from build123d import *

# Parameters (mm, degrees)
F0_W     = 914.4
F0_H     = 330.2
F2_DEPTH = 19.05
F1_R     = 139.7
F3_DEPTH = 982
F4_DEPTH = 19.051
F5_R     = 139.7
F6_DEPTH = 19.051


# Not quite as in the source:
# - an extrude ends at something that could not be found from the text; its depth is read off the source's solid


with BuildPart() as f2:
    # F0 (on Front) → F2 (new body)
    with BuildSketch(Plane.XZ):
        Rectangle(F0_W, F0_H)
    extrude(amount=F2_DEPTH)

    # F1 (on face) → F3 (cut, through all)
    with BuildSketch(Plane.XZ):
        with Locations((-228.6, 0)):
            Circle(F1_R)
    extrude(amount=-F3_DEPTH, mode=Mode.SUBTRACT)

    # F1 (on face) → F4 (cut, through all)
    with BuildSketch(Plane.XZ):
        with Locations((-228.6, 0)):
            Circle(F1_R)
    extrude(amount=F4_DEPTH, mode=Mode.SUBTRACT)

    # F5 (on face) → F6 (cut, through all)
    with BuildSketch(Plane.XZ.offset(19.05)):
        with Locations((228.6, 0)):
            Circle(F5_R)
    extrude(amount=-F6_DEPTH, mode=Mode.SUBTRACT)


solid = f2.part
Verification items for the finished model (mm, model axes). Coordinates: 2 decimals unless noted, no trailing zeros. Order: outer loops, then holes, each group sorted by start corner. A loop starts at its lowest first (then second) coordinate and runs counter-clockwise, first axis right, second up. Notation, with made-up numbers: (4, 45) -> (23, 45) arc R22 ccw to (23, 77) -> close; hole circle Ø8 at (28.5, 53). An arc over 180 degrees is marked (long way). Use CSV: the item, a comma, the result in double quotes. Start each with the question number.
Q1. Thickness scan on line 1 along Z through (x, y) = (-228.6, -4.5); line 2 along X through (y, z) = (-10, -90); line 3 along X through (y, z) = (-8.75, 13.5). Record the ranges inside material, lowest first.
Q2. Section check D-D, the plane z = 38. Record the cut outline in (x, y), and give its area (3 significant figures).
Q3. Section check A-A, the plane x = -228.6. Record the cut outline in (y, z), and give its area (3 significant figures).
Q4. Section check B-B, the plane z = 0. Record the cut outline in (x, y), and give its area (3 significant figures).
Q5. Section check C-C, the plane y = -14. Record the cut outline in (x, z), and give its area (3 significant figures).
Q6. Draft check along Z on faces 1 (the flat face through (-6, -19.05, 2)), 2 (the cylindrical face through (-368.165, -9.392, 6.142)), 3 (the flat face through (-6, -9, -165.1)). Enter one of: +Z half, -Z half, draft (parallel to the pull), parting line (faces both ways), or undercut.
Returned:
1,line 1,"z = -165.1 to -139.7, 139.7 to 165.1"
1,line 2,"x = -457.2 to -335.45, -121.75 to 121.75, 335.45 to 457.2"
1,line 3,"x = -457.2 to -367.65, -89.55 to 89.55, 367.65 to 457.2"
2,outline,"(-457.2, -19.05) -> (-363.03, -19.05) -> (-363.03, 0) -> (-457.2, 0) -> close; (-94.17, -19.05) -> (94.17, -19.05) -> (94.17, 0) -> (-94.17, 0) -> close; (363.03, -19.05) -> (457.2, -19.05) -> (457.2, 0) -> (363.03, 0) -> close"
2,area,"7,180 mm^2"
3,outline,"(-19.05, -165.1) -> (0, -165.1) -> (0, -139.7) -> (-19.05, -139.7) -> close; (-19.05, 139.7) -> (0, 139.7) -> (0, 165.1) -> (-19.05, 165.1) -> close"
3,area,"968 mm^2"
4,outline,"(-457.2, -19.05) -> (-368.3, -19.05) -> (-368.3, 0) -> (-457.2, 0) -> close; (-88.9, -19.05) -> (88.9, -19.05) -> (88.9, 0) -> (-88.9, 0) -> close; (368.3, -19.05) -> (457.2, -19.05) -> (457.2, 0) -> (368.3, 0) -> close"
4,area,"6,770 mm^2"
5,outline,"(-457.2, -165.1) -> (457.2, -165.1) -> (457.2, 165.1) -> (-457.2, 165.1) -> close; hole circle Ø279.4 at (-228.6, 0); hole circle Ø279.4 at (228.6, 0)"
5,area,"179,000 mm^2"
6,face 1,"draft"
6,face 2,"undercut"
6,face 3,"-Z half"
